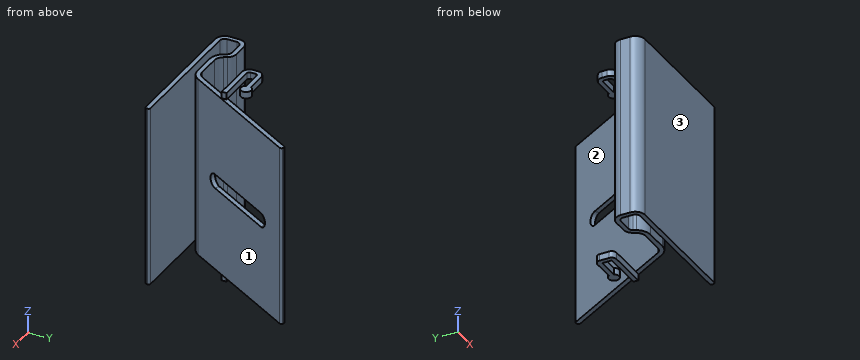
```python
from build123d import *

# Parameters (mm, degrees)
EXTRUDE_12_DEPTH    = 190
CUT_EXTRUDE_1_REACH = 78.573
SKETCH_3_12_R       = 5.5
EXTRUDE_13_DEPTH    = 7
EXTRUDE_14_DEPTH    = 7
EXTRUDE_16_DEPTH    = 7


with BuildPart() as part:
    # Sketch 3 → Extrude 12 (new body)
    with BuildSketch(Plane.XY):
        with BuildLine():
            ThreePointArc((74, 128.17175976), (75.214412717, 129.103611413), (76.732050808, 128.903810568))
            Line((76.732050808, 128.903810568), (77.598076211, 128.403810568))
            ThreePointArc((77.598076211, 128.403810568), (78.529927864, 127.18939785), (78.330127019, 125.67175976))
            Line((78.330127019, 125.67175976), (7.216878365, 2.5))
            ThreePointArc((7.216878365, 2.5), (1.726497308, -2.990381057), (-5.773502692, -5))
            Line((-5.773502692, -5), (-29.226497308, -5))
            ThreePointArc((-29.226497308, -5), (-36.726497308, -2.990381057), (-42.216878365, 2.5))
            Line((-42.216878365, 2.5), (-43.943375673, 5.490381057))
            ThreePointArc((-43.943375673, 5.490381057), (-45.773502692, 7.320508076), (-48.273502692, 7.990381057))
            Line((-48.273502692, 7.990381057), (-62.5, 7.990381057))
            ThreePointArc((-62.5, 7.990381057), (-66.035533906, 6.525914963), (-67.5, 2.990381057))
            Line((-67.5, 2.990381057), (-67.5, -7.009618943))
            ThreePointArc((-67.5, -7.009618943), (-66.035533906, -10.545152849), (-62.5, -12.009618943))
            Line((-62.5, -12.009618943), (73, -12.009618943))
            ThreePointArc((73, -12.009618943), (74.414213562, -12.595405381), (75, -14.009618943))
            Line((75, -14.009618943), (75, -15.009618943))
            ThreePointArc((75, -15.009618943), (74.414213562, -16.423832506), (73, -17.009618943))
            Line((73, -17.009618943), (-62.5, -17.009618943))
            ThreePointArc((-62.5, -17.009618943), (-69.571067812, -14.080686755), (-72.5, -7.009618943))
            Line((-72.5, -7.009618943), (-72.5, 2.990381057))
            ThreePointArc((-72.5, 2.990381057), (-69.571067812, 10.061448869), (-62.5, 12.990381057))
            Line((-62.5, 12.990381057), (-48.273502692, 12.990381057))
            ThreePointArc((-48.273502692, 12.990381057), (-43.273502692, 11.650635095), (-39.613248654, 7.990381057))
            Line((-39.613248654, 7.990381057), (-37.886751346, 5))
            ThreePointArc((-37.886751346, 5), (-34.226497308, 1.339745962), (-29.226497308, 0))
            Line((-29.226497308, 0), (-5.773502692, 0))
            ThreePointArc((-5.773502692, 0), (-0.773502692, 1.339745962), (2.886751346, 5))
            Line((2.886751346, 5), (74, 128.17175976))
        make_face()
    extrude(amount=-EXTRUDE_12_DEPTH)

    # Sketch 19 → Cut-Extrude 1 (cut, up to next)
    with BuildSketch(Plane(origin=(0, 0, 0), x_dir=(0, 0, 1), z_dir=(-0.866025404, 0.5, 0)), mode=Mode.PRIVATE) as cut_extrude_1_sk1:
        with BuildLine():
            Line((-95, 107.5), (-95, 115))
            Line((-95, 115), (-102.5, 115))
            ThreePointArc((-102.5, 115), (-100.303300859, 109.696699141), (-95, 107.5))
        make_face()
    cut_extrude_1_tool1 = extrude(cut_extrude_1_sk1.sketch, amount=-CUT_EXTRUDE_1_REACH, mode=Mode.PRIVATE) & part.part
    add(cut_extrude_1_tool1.solids().sort_by_distance((55.908451, 96.836277, -98.183099))[0], mode=Mode.SUBTRACT)
    # Sketch 19 → Cut-Extrude 1 (cut, up to next)
    with BuildSketch(Plane(origin=(0, 0, 0), x_dir=(0, 0, 1), z_dir=(-0.866025404, 0.5, 0)), mode=Mode.PRIVATE) as cut_extrude_1_sk2:
        with BuildLine():
            Line((-87.5, 115), (-95, 115))
            Line((-95, 115), (-95, 107.5))
            ThreePointArc((-95, 107.5), (-89.696699141, 109.696699141), (-87.5, 115))
        make_face()
    cut_extrude_1_tool2 = extrude(cut_extrude_1_sk2.sketch, amount=-CUT_EXTRUDE_1_REACH, mode=Mode.PRIVATE) & part.part
    add(cut_extrude_1_tool2.solids().sort_by_distance((55.908451, 96.836277, -91.816901))[0], mode=Mode.SUBTRACT)
    # Sketch 19 → Cut-Extrude 1 (cut, up to next)
    with BuildSketch(Plane(origin=(0, 0, 0), x_dir=(0, 0, 1), z_dir=(-0.866025404, 0.5, 0)), mode=Mode.PRIVATE) as cut_extrude_1_sk3:
        with BuildLine():
            Line((-102.5, 115), (-95, 115))
            Line((-95, 115), (-87.5, 115))
            ThreePointArc((-87.5, 115), (-95, 122.5), (-102.5, 115))
        make_face()
    cut_extrude_1_tool3 = extrude(cut_extrude_1_sk3.sketch, amount=-CUT_EXTRUDE_1_REACH, mode=Mode.PRIVATE) & part.part
    add(cut_extrude_1_tool3.solids().sort_by_distance((59.091549, 102.349566, -95))[0], mode=Mode.SUBTRACT)
    # Sketch 19 → Cut-Extrude 1 (cut, up to next)
    with BuildSketch(Plane(origin=(0, 0, 0), x_dir=(0, 0, 1), z_dir=(-0.866025404, 0.5, 0)), mode=Mode.PRIVATE) as cut_extrude_1_sk4:
        with BuildLine():
            ThreePointArc((-95, 107.5), (-100.303300859, 109.696699141), (-102.5, 115))
            Line((-102.5, 115), (-102.5, 35))
            ThreePointArc((-102.5, 35), (-100.303300859, 40.303300859), (-95, 42.5))
            Line((-95, 42.5), (-95, 107.5))
        make_face()
    cut_extrude_1_tool4 = extrude(cut_extrude_1_sk4.sketch, amount=-CUT_EXTRUDE_1_REACH, mode=Mode.PRIVATE) & part.part
    add(cut_extrude_1_tool4.solids().sort_by_distance((37.5, 64.951905, -98.8479))[0], mode=Mode.SUBTRACT)
    # Sketch 19 → Cut-Extrude 1 (cut, up to next)
    with BuildSketch(Plane(origin=(0, 0, 0), x_dir=(0, 0, 1), z_dir=(-0.866025404, 0.5, 0)), mode=Mode.PRIVATE) as cut_extrude_1_sk5:
        with BuildLine():
            ThreePointArc((-87.5, 115), (-89.696699141, 109.696699141), (-95, 107.5))
            Line((-95, 107.5), (-95, 42.5))
            ThreePointArc((-95, 42.5), (-89.696699141, 40.303300859), (-87.5, 35))
            Line((-87.5, 35), (-87.5, 115))
        make_face()
    cut_extrude_1_tool5 = extrude(cut_extrude_1_sk5.sketch, amount=-CUT_EXTRUDE_1_REACH, mode=Mode.PRIVATE) & part.part
    add(cut_extrude_1_tool5.solids().sort_by_distance((37.5, 64.951905, -91.1521))[0], mode=Mode.SUBTRACT)
    # Sketch 19 → Cut-Extrude 1 (cut, up to next)
    with BuildSketch(Plane(origin=(0, 0, 0), x_dir=(0, 0, 1), z_dir=(-0.866025404, 0.5, 0)), mode=Mode.PRIVATE) as cut_extrude_1_sk6:
        with BuildLine():
            ThreePointArc((-95, 42.5), (-100.303300859, 40.303300859), (-102.5, 35))
            Line((-102.5, 35), (-95, 35))
            Line((-95, 35), (-95, 42.5))
        make_face()
    cut_extrude_1_tool6 = extrude(cut_extrude_1_sk6.sketch, amount=-CUT_EXTRUDE_1_REACH, mode=Mode.PRIVATE) & part.part
    add(cut_extrude_1_tool6.solids().sort_by_distance((19.091549, 33.067534, -98.183099))[0], mode=Mode.SUBTRACT)
    # Sketch 19 → Cut-Extrude 1 (cut, up to next)
    with BuildSketch(Plane(origin=(0, 0, 0), x_dir=(0, 0, 1), z_dir=(-0.866025404, 0.5, 0)), mode=Mode.PRIVATE) as cut_extrude_1_sk7:
        with BuildLine():
            Line((-95, 35), (-102.5, 35))
            ThreePointArc((-102.5, 35), (-95, 27.5), (-87.5, 35))
            Line((-87.5, 35), (-95, 35))
        make_face()
    cut_extrude_1_tool7 = extrude(cut_extrude_1_sk7.sketch, amount=-CUT_EXTRUDE_1_REACH, mode=Mode.PRIVATE) & part.part
    add(cut_extrude_1_tool7.solids().sort_by_distance((15.908451, 27.554245, -95))[0], mode=Mode.SUBTRACT)
    # Sketch 19 → Cut-Extrude 1 (cut, up to next)
    with BuildSketch(Plane(origin=(0, 0, 0), x_dir=(0, 0, 1), z_dir=(-0.866025404, 0.5, 0)), mode=Mode.PRIVATE) as cut_extrude_1_sk8:
        with BuildLine():
            ThreePointArc((-87.5, 35), (-89.696699141, 40.303300859), (-95, 42.5))
            Line((-95, 42.5), (-95, 35))
            Line((-95, 35), (-87.5, 35))
        make_face()
    cut_extrude_1_tool8 = extrude(cut_extrude_1_sk8.sketch, amount=-CUT_EXTRUDE_1_REACH, mode=Mode.PRIVATE) & part.part
    add(cut_extrude_1_tool8.solids().sort_by_distance((19.091549, 33.067534, -91.816901))[0], mode=Mode.SUBTRACT)



with BuildPart() as body_2:
    # Sketch 3_12 → Extrude 13 (new body)
    with BuildSketch(Plane.XY):
        with Locations((11.547005384, 55)):
            Circle(SKETCH_3_12_R)
    extrude(amount=EXTRUDE_13_DEPTH)


with BuildPart() as part_1:
    add(part.part)

    add(body_2.part)  # Extrude 14 merges body 2
    # Sketch 20 → Extrude 14 (add)
    with BuildSketch(Plane.XY):
        with BuildLine():
            Line((-13.452994616, 55), (11.547005384, 55))
            Line((11.547005384, 55), (11.547005384, 57.5))
            Line((11.547005384, 57.5), (-13.452994616, 57.5))
            ThreePointArc((-13.452994616, 57.5), (-18.756295475, 55.303300859), (-20.952994616, 50))
            Line((-20.952994616, 50), (-20.952994616, 45))
            ThreePointArc((-20.952994616, 45), (-18.756295475, 39.696699141), (-13.452994616, 37.5))
            Line((-13.452994616, 37.5), (26.547005384, 37.5))
            Line((26.547005384, 37.5), (26.547005384, 40))
            Line((26.547005384, 40), (-13.452994616, 40))
            ThreePointArc((-13.452994616, 40), (-16.988528522, 41.464466094), (-18.452994616, 45))
            Line((-18.452994616, 45), (-18.452994616, 50))
            ThreePointArc((-18.452994616, 50), (-16.988528522, 53.535533906), (-13.452994616, 55))
        make_face()
        with BuildLine():
            Line((11.547005384, 52.5), (11.547005384, 55))
            Line((11.547005384, 55), (-13.452994616, 55))
            ThreePointArc((-13.452994616, 55), (-16.988528522, 53.535533906), (-18.452994616, 50))
            Line((-18.452994616, 50), (-18.452994616, 45))
            ThreePointArc((-18.452994616, 45), (-16.988528522, 41.464466094), (-13.452994616, 40))
            Line((-13.452994616, 40), (26.547005384, 40))
            Line((26.547005384, 40), (26.547005384, 42.5))
            Line((26.547005384, 42.5), (-13.452994616, 42.5))
            ThreePointArc((-13.452994616, 42.5), (-15.220761569, 43.232233047), (-15.952994616, 45))
            Line((-15.952994616, 45), (-15.952994616, 50))
            ThreePointArc((-15.952994616, 50), (-15.220761569, 51.767766953), (-13.452994616, 52.5))
            Line((-13.452994616, 52.5), (11.547005384, 52.5))
        make_face()
    extrude(amount=EXTRUDE_14_DEPTH)

    # Sketch 21 → Extrude 16 (add)
    with BuildSketch(Plane(origin=(0, 0, -190), x_dir=(-1, 0, 0), z_dir=(0, 0, -1))):
        with BuildLine():
            Line((-11.547005384, 52.5), (-11.547005384, 55))
            Line((-11.547005384, 55), (-11.547005384, 57.5))
            Line((-11.547005384, 57.5), (-6.648025898, 57.5))
            ThreePointArc((-6.648025898, 57.5), (-17.047005384, 55), (-6.648025898, 52.5))
            Line((-6.648025898, 52.5), (-11.547005384, 52.5))
        make_face()
        with BuildLine():
            Line((-11.547005384, 57.5), (-11.547005384, 55))
            Line((-11.547005384, 55), (-6.047005384, 55))
            ThreePointArc((-6.047005384, 55), (-6.199370992, 56.285615189), (-6.648025898, 57.5))
            Line((-6.648025898, 57.5), (-11.547005384, 57.5))
        make_face()
        with BuildLine():
            Line((-6.047005384, 55), (-11.547005384, 55))
            Line((-11.547005384, 55), (-11.547005384, 52.5))
            Line((-11.547005384, 52.5), (-6.648025898, 52.5))
            ThreePointArc((-6.648025898, 52.5), (-6.199370992, 53.714384811), (-6.047005384, 55))
        make_face()
        with BuildLine():
            ThreePointArc((-6.648025898, 57.5), (-6.199370992, 56.285615189), (-6.047005384, 55))
            Line((-6.047005384, 55), (15.952994616, 55))
            ThreePointArc((15.952994616, 55), (17.720761569, 54.267766953), (18.452994616, 52.5))
            Line((18.452994616, 52.5), (18.452994616, 42.5))
            ThreePointArc((18.452994616, 42.5), (17.720761569, 40.732233047), (15.952994616, 40))
            Line((15.952994616, 40), (-23.094010768, 40))
            Line((-23.094010768, 40), (-21.650635095, 37.5))
            Line((-21.650635095, 37.5), (15.952994616, 37.5))
            ThreePointArc((15.952994616, 37.5), (19.488528522, 38.964466094), (20.952994616, 42.5))
            Line((20.952994616, 42.5), (20.952994616, 52.5))
            ThreePointArc((20.952994616, 52.5), (19.488528522, 56.035533906), (15.952994616, 57.5))
            Line((15.952994616, 57.5), (-6.648025898, 57.5))
        make_face()
        with BuildLine():
            Line((15.952994616, 55), (-6.047005384, 55))
            ThreePointArc((-6.047005384, 55), (-6.199370992, 53.714384811), (-6.648025898, 52.5))
            Line((-6.648025898, 52.5), (15.952994616, 52.5))
            Line((15.952994616, 52.5), (15.952994616, 42.5))
            Line((15.952994616, 42.5), (-24.537386441, 42.5))
            Line((-24.537386441, 42.5), (-23.094010768, 40))
            Line((-23.094010768, 40), (15.952994616, 40))
            ThreePointArc((15.952994616, 40), (17.720761569, 40.732233047), (18.452994616, 42.5))
            Line((18.452994616, 42.5), (18.452994616, 52.5))
            ThreePointArc((18.452994616, 52.5), (17.720761569, 54.267766953), (15.952994616, 55))
        make_face()
        Polygon((-23.094010768, 40), (-24.537386441, 42.5), (-26.547005384, 42.5), (-26.547005384, 40), align=None)
        Polygon((-21.650635095, 37.5), (-23.094010768, 40), (-26.547005384, 40), (-26.547005384, 37.5), align=None)
    extrude(amount=EXTRUDE_16_DEPTH)


solid = part_1.part
```
Check sheet for the modelled part. Datum: model origin and axes. Units: mm. Face numbers are marked on the shaded views. Coordinates: 2 decimals unless noted, no trailing zeros. Order: outer loops, then holes, each group sorted by start corner. A loop starts at its lowest first (then second) coordinate and runs counter-clockwise, first axis right, second up. Notation, with made-up numbers: (63.5, 74) -> (106.5, 74) arc R19 ccw to (106.5, 98) -> close; hole circle Ø1 at (-1, 56). An arc over 180 degrees is marked (long way). Write each question's results on one line, items separated by ' | '. Start each with the question number.
1) Section check A-A (z = -151). Enter the section's corners in (x, y).
2) Material ranges on line 1 along Y through (x, z) = (-20, -181.5); line 2 along X through (y, z) = (-7, -45); line 3 along Y through (x, z) = (-4, -134), recorded low to high.
3) Depth check by flat-ended pin: pin 1 (2 mm diameter, centred on x = 0, z = -194.5, fed in from -Y); pin 2 (3 mm diameter, centred on x = 54.5, z = -15.5, fed in from +Y); pin 3 (1 mm diameter, centred on y = 93, z = -14.5, fed in from +X). Enter the tip coordinate at first touch or a pass-through.
4) Section check C-C (y = 72). Enter the section's corners in (x, z), and give its area (3 significant figures).
5) Draft check along Y on the marked faces 1, 2 and 3. Enter one of: pulls with the +Y half, pulls with the -Y half, needs draft (parallel to the pull), parting line crosses it, or undercut.
6) Section check B-B (y = 55). Enter the section's corners in (x, z), and give its area (3 significant figures).
7) Section check D-D (y = 17.5). Enter the section's corners in (x, z).
Checked values:
1) outline: (-72.5, -7.01) arc R10 ccw to (-62.5, -17.01) -> (73, -17.01) arc R2 ccw to (75, -15.01) -> (75, -14.01) arc R2 ccw to (73, -12.01) -> (-62.5, -12.01) arc R5 cw to (-67.5, -7.01) -> (-67.5, 2.99) arc R5 cw to (-62.5, 7.99) -> (-48.27, 7.99) arc R5 cw to (-43.94, 5.49) -> (-42.22, 2.5) arc R15 ccw to (-29.23, -5) -> (-5.77, -5) arc R15 ccw to (7.22, 2.5) -> (78.33, 125.67) arc R2 ccw to (77.6, 128.4) -> (76.73, 128.9) arc R2 ccw to (74, 128.17) -> (2.89, 5) arc R10 cw to (-5.77, 0) -> (-29.23, 0) arc R10 cw to (-37.89, 5) -> (-39.61, 7.99) arc R10 ccw to (-48.27, 12.99) -> (-62.5, 12.99) arc R10 ccw to (-72.5, 2.99) -> close
2) line 1: -17.01 to -12.01, -5 to 0 | line 2: -72.5 to -67.5 | line 3: -17.01 to -12.01, -4.89 to 0.16
3) pin 1: y = 37.5 | pin 2: y = 96.99 | pin 3: x = 59.76
4) outline: (41.57, -190) -> (47.34, -190) -> (47.34, -102.5) -> (41.57, -102.5) -> close; (41.57, -87.5) -> (47.34, -87.5) -> (47.34, 0) -> (41.57, 0) -> close | area: 1,010 mm²
5) face 1: undercut | face 2: pulls with the +Y half | face 3: pulls with the -Y half
6) outline: (-20.28, -197) -> (17.05, -197) -> (17.05, -190) -> (-20.28, -190) -> close; (-19.04, 0) -> (17.05, 0) -> (17.05, 7) -> (-19.04, 7) -> close; (31.75, -190) -> (37.53, -190) -> (37.53, -102.5) -> (31.75, -102.5) -> close; (31.75, -87.5) -> (37.53, -87.5) -> (37.53, 0) -> (31.75, 0) -> close | area: 1,520 mm²
7) outline: (10.1, -190) -> (15.88, -190) -> (15.88, 0) -> (10.1, 0) -> close
